The model under review builds one solid part; all positions refer to its coordinate system, in mm. A direction names the side the tool comes from. Give positions to 0.01 mm unless a question says otherwise; leave off trailing zeros. Write each loop counter-clockwise with the first axis right and the second up, starting at its lowest first coordinate (ties: lowest second). Pieces come first, ordered by that corner, then holes.
from build123d import *

# Parameters (mm, degrees)
F2_DEPTH = 2.5
F4_SIZE  = 1
F5_SIZE  = 1


with BuildPart() as f2:
    # F1 (on face) → F2 (new body)
    with BuildSketch(Plane.XY):
        Polygon((-8, -1), (-18, -1), (-18, -5), (-5.5, -5), (-0.3375368448, 2), (0, 2), (0, 7), (-1.1940948898, 7), align=None)
    extrude(amount=F2_DEPTH)

    # F3: F2 across plane


with BuildPart() as f2_1:
    add(f2.part)
    add(f2.part.mirror(Plane.YZ))

    # F4 (call 1 of 3: OpenCascade refuses the feature's edges together)
    f4_edges = [f2_1.edges().sort_by_distance(p)[0] for p in [
        (-11.75, -5, 2.5),
        (-2.918768, -1.5, 2.5),
        (2.918768, -1.5, 2.5),
        (11.75, -5, 2.5),
        (0, 2, 2.5),
    ]]
    chamfer(f4_edges, length=F4_SIZE)

    # F4#2 (call 2 of 3)
    f4_2_edges = [f2_1.edges().sort_by_distance(p)[0] for p in [
        (-13, -1, 2.5),
        (-4.597047, 3, 2.5),
    ]]
    chamfer(f4_2_edges, length=F4_SIZE)

    # F4#3 (call 3 of 3)
    f4_3_edges = [f2_1.edges().sort_by_distance(p)[0] for p in [
        (4.597047, 3, 2.5),
        (13, -1, 2.5),
    ]]
    chamfer(f4_3_edges, length=F4_SIZE)

    # F5
    f5_edges = [f2_1.edges().sort_by_distance(p)[0] for p in [
        (0, 6.930164, 2.454748),
    ]]
    chamfer(f5_edges, length=F5_SIZE)


solid = f2_1.part
1) Insertion check: pin 1 (0.8 mm diameter, centred on x = -12.5, z = 0.5, fed in from +Y). The pin has a flat end and moves straight along its axis. Give the tip position at first contact, or say it passes through.
2) To check wall thickness, follow probe 1 along Y at (x, z) = (16, 1.4); probe 2 along X at (y, z) = (0, 0.9); probe 3 along X at (y, z) = (-3.5, 0.6). State the ranges of each line that lie inside material, in increasing order.
3) Tool access review of faces 1 (the flat face through (2.955, -1.549, 0.74)), 2 (the flat face through (13, -1, 1)), 3 (the flat face through (0, 2.6, 2.1)): name each direction out of +Z, -Z, +X, -X, +Y, -Y from which nothing blocks a thin tool from reaching the whole face with its end or side.
4) Consider section B-B, the plane x = 15. Give the boundary of the cut face in (y, z), then the cut area to 3 significant figures.
5) Consider section C-C, the plane y = -3.5. Give the boundary of the cut face in (x, z).
6) Consider section D-D, the plane x = 4.5. Give the boundary of the cut face in (y, z).
7) Consider section A-A, the plane z = 0.7. Give the boundary of the cut face in (x, y).
8) The part is to be moulded in two halves that separate along X. For faces 4 (the flat face through (-2.955, -1.549, 0.74)), 5 (the flat face through (4.25, 2.65, 1.99)), 6 (the flat face through (0, 7, 1)), say which applies: +X half, -X half, draft (parallel to the pull), parting line (faces both ways), or undercut.
Answer block:
1. pin 1: stops at y = -1
2. probe 1: y = -5 to -1
2. probe 2: x = -7.15 to -1.81, 1.81 to 7.15
2. probe 3: x = -18 to -4.39, 4.39 to 18
3. face 1: +Z, -Z, -Y
3. face 2: +Z, -Z, +X, +Y
3. face 3: +Z, -Y
4. outline: (-5, 0) - (-1, 0) - (-1, 1.5) - (-2, 2.5) - (-4, 2.5) - (-5, 1.5) - close
4. area: 9.00 mm2
5. outline: (-18, 0) - (-4.39, 0) - (-4.39, 1.5) - (-5.64, 2.5) - (-18, 2.5) - close; (4.39, 0) - (18, 0) - (18, 2.5) - (5.64, 2.5) - (4.39, 1.5) - close
6. outline: (-3.64, 0) - (3.11, 0) - (3.11, 1.5) - (1.57, 2.5) - (-1.96, 2.5) - (-3.64, 1.5) - close
7. outline: (-18, -5) - (-5.5, -5) - (-0.34, 2) - (0.34, 2) - (5.5, -5) - (18, -5) - (18, -1) - (8, -1) - (1.19, 7) - (-1.19, 7) - (-8, -1) - (-18, -1) - close
8. face 4: undercut
8. face 5: +X half
8. face 6: draft
